```python
from build123d import *

# Parameters (mm, degrees)
SALIENTE_EXTRUIR1_DEPTH = 2.5
SALIENTE_EXTRUIR2_START = 90
SALIENTE_EXTRUIR2_DEPTH = 90
CORTAR_EXTRUIR2_REACH   = 171.292
CORTAR_EXTRUIR4_DEPTH   = 63
REDONDEO1_R             = 1
CORTAR_EXTRUIR5_REACH   = 171.292
CROQUIS7_R              = 1.5
CORTAR_EXTRUIR6_DEPTH   = 5


with BuildPart() as part:
    # Croquis1 → Saliente-Extruir1 (new body)
    with BuildSketch(Plane(origin=(0, 95.6, 0), x_dir=(1, 0, 0), z_dir=(0, 1, 0))):
        with BuildLine():
            Line((327.757359313, -46.5), (227.242640687, -46.5))
            Line((227.242640687, -46.5), (217.1, -46.5))
            ThreePointArc((217.1, -46.5), (214.271572875, -45.328427125), (213.1, -42.5))
            Line((213.1, -42.5), (213.1, 42.5))
            ThreePointArc((213.1, 42.5), (214.271572875, 45.328427125), (217.1, 46.5))
            Line((217.1, 46.5), (227.242640687, 46.5))
            Line((227.242640687, 46.5), (327.757359313, 46.5))
            ThreePointArc((327.757359313, 46.5), (331.966877069, 45.662674858), (335.535533906, 43.278174593))
            Line((335.535533906, 43.278174593), (339.778174891, 39.035533608))
            ThreePointArc((339.778174891, 39.035533608), (342.162674938, 35.466876874), (343, 31.257359313))
            Line((343, 31.257359313), (343, -31.257359312))
            ThreePointArc((343, -31.257359312), (342.162674858, -35.466877069), (339.778174593, -39.035533906))
            Line((339.778174593, -39.035533906), (335.535533608, -43.278174891))
            ThreePointArc((335.535533608, -43.278174891), (331.966876874, -45.662674939), (327.757359313, -46.5))
        make_face()
    extrude(amount=SALIENTE_EXTRUIR1_DEPTH)

    # Croquis2 → Saliente-Extruir2 (add)
    with BuildSketch(Plane.XZ.offset(-95.6).offset(SALIENTE_EXTRUIR2_START)):
        with BuildLine():
            Line((213.1, 42.5), (213.1, -42.5))
            ThreePointArc((213.1, -42.5), (214.271572875, -45.328427125), (217.1, -46.5))
            Line((217.1, -46.5), (327.757359313, -46.5))
            ThreePointArc((327.757359313, -46.5), (331.966877069, -45.662674858), (335.535533906, -43.278174593))
            Line((335.535533906, -43.278174593), (339.778174891, -39.035533608))
            ThreePointArc((339.778174891, -39.035533608), (342.162674938, -35.466876874), (343, -31.257359313))
            Line((343, -31.257359313), (343, 31.257359312))
            ThreePointArc((343, 31.257359312), (342.162674858, 35.466877069), (339.778174593, 39.035533906))
            Line((339.778174593, 39.035533906), (335.535533608, 43.278174891))
            ThreePointArc((335.535533608, 43.278174891), (331.966876874, 45.662674939), (327.757359313, 46.5))
            Line((327.757359313, 46.5), (217.1, 46.5))
            ThreePointArc((217.1, 46.5), (214.271572875, 45.328427125), (213.1, 42.5))
        make_face()
        with BuildLine():
            Line((220.6, 39), (220.6, -39))
            Line((220.6, -39), (327.757359313, -39))
            ThreePointArc((327.757359313, -39), (329.096751326, -38.733578364), (330.232233047, -37.974873734))
            Line((330.232233047, -37.974873734), (334.474874032, -33.732232749))
            ThreePointArc((334.474874032, -33.732232749), (335.233578444, -32.596751131), (335.5, -31.257359313))
            Line((335.5, -31.257359313), (335.5, 31.257359312))
            ThreePointArc((335.5, 31.257359312), (335.233578364, 32.596751326), (334.474873734, 33.732233047))
            Line((334.474873734, 33.732233047), (330.232232749, 37.974874033))
            ThreePointArc((330.232232749, 37.974874033), (329.096751131, 38.733578445), (327.757359313, 39))
            Line((327.757359313, 39), (220.6, 39))
        make_face(mode=Mode.SUBTRACT)
    extrude(amount=-SALIENTE_EXTRUIR2_DEPTH)

    # Croquis3 → Cortar-Extruir2 (cut, up to next)
    with BuildSketch(Plane(origin=(343, 0, 0), x_dir=(0, 0, -1), z_dir=(1, 0, 0)), mode=Mode.PRIVATE) as cortar_extruir2_sk1:
        with BuildLine():
            Line((23, 85.4), (-24.5, 85.4))
            ThreePointArc((-24.5, 85.4), (-27.540559159, 84.140559159), (-28.8, 81.1))
            Line((-28.8, 81.1), (-28.8, 40.6))
            ThreePointArc((-28.8, 40.6), (-27.101219331, 36.498780669), (-23, 34.8))
            Line((-23, 34.8), (24.5, 34.8))
            ThreePointArc((24.5, 34.8), (27.540559159, 36.059440841), (28.8, 39.1))
            Line((28.8, 39.1), (28.8, 79.6))
            ThreePointArc((28.8, 79.6), (27.101219331, 83.701219331), (23, 85.4))
        make_face()
    cortar_extruir2_tool1 = extrude(cortar_extruir2_sk1.sketch, amount=-CORTAR_EXTRUIR2_REACH, mode=Mode.PRIVATE) & part.part
    add(cortar_extruir2_tool1.solids().sort_by_distance((343, 60.1, 0))[0], mode=Mode.SUBTRACT)

    # Croquis4 → Cortar-Extruir4 (cut)
    with BuildSketch(Plane(origin=(0, 98.1, 0), x_dir=(1, 0, 0), z_dir=(0, 1, 0))):
        Polygon((232.757359313, -33.9), (232.757359313, -38.5), (232.757359313, -46.5), (326.657359313, -46.5), (326.657359313, -38.5), (326.657359313, -33.9), align=None)
        Polygon((326.657359313, 46.5), (232.757359313, 46.5), (232.757359313, 38.5), (232.757359313, 33.9), (326.657359313, 33.9), (326.657359313, 38.5), align=None)
    extrude(amount=-CORTAR_EXTRUIR4_DEPTH, mode=Mode.SUBTRACT)

    # Redondeo1
    redondeo1_edges = [part.edges().sort_by_distance(p)[0] for p in [
        (232.757359313, 95.6, -36.45),
        (279.707359313, 95.6, -33.9),
        (326.657359313, 95.6, -36.45),
        (279.707359313, 95.6, 33.9),
        (232.757359313, 95.6, 36.45),
        (326.657359313, 95.6, 36.45),
        (279.707359313, 35.1, 39),
        (279.707359313, 35.1, -39),
        (326.657359313, 65.35, 39),
        (232.757359313, 65.35, 39),
        (232.757359313, 96.85, 33.9),
        (326.657359313, 96.85, 33.9),
        (326.657359313, 35.1, 42.75),
        (279.707359313, 35.1, 46.5),
        (326.657359313, 66.6, 46.5),
        (232.757359313, 35.1, 42.75),
        (232.757359313, 66.6, 46.5),
        (326.657359313, 98.1, 40.2),
        (279.707359313, 98.1, 33.9),
        (232.757359313, 98.1, 40.2),
        (326.657359313, 65.35, -39),
        (326.657359313, 96.85, -33.9),
        (232.757359313, 65.35, -39),
        (326.657359313, 35.1, -42.75),
        (326.657359313, 66.6, -46.5),
        (232.757359313, 96.85, -33.9),
        (232.757359313, 35.1, -42.75),
        (279.707359313, 35.1, -46.5),
        (232.757359313, 66.6, -46.5),
        (326.657359313, 98.1, -40.2),
        (232.757359313, 98.1, -40.2),
        (279.707359313, 98.1, -33.9),
    ]]
    fillet(redondeo1_edges, radius=REDONDEO1_R)

    # Croquis5 → Cortar-Extruir5 (cut, up to next)
    with BuildSketch(Plane.ZY.offset(-213.1), mode=Mode.PRIVATE) as cortar_extruir5_sk1:
        with BuildLine():
            Line((-19.675765155, 71.72423484), (-19.675765155, 48.475765161))
            ThreePointArc((-19.675765155, 48.475765161), (-21.433124468, 44.233124467), (-25.675765163, 42.475765155))
            Line((-25.675765163, 42.475765155), (-31.024234836, 42.475765155))
            ThreePointArc((-31.024234836, 42.475765155), (-35.266875531, 44.233124467), (-37.024234845, 48.475765162))
            Line((-37.024234845, 48.475765162), (-37.024234845, 71.724234837))
            ThreePointArc((-37.024234845, 71.724234837), (-35.266875532, 75.966875532), (-31.024234837, 77.724234845))
            Line((-31.024234837, 77.724234845), (-25.675765164, 77.724234845))
            ThreePointArc((-25.675765164, 77.724234845), (-21.433124469, 75.966875534), (-19.675765155, 71.72423484))
        make_face()
    cortar_extruir5_tool1 = extrude(cortar_extruir5_sk1.sketch, amount=-CORTAR_EXTRUIR5_REACH, mode=Mode.PRIVATE) & part.part
    add(cortar_extruir5_tool1.solids().sort_by_distance((213.1, 60.1, -28.35))[0], mode=Mode.SUBTRACT)

    # Croquis7 → Cortar-Extruir6 (cut)
    with BuildSketch(Plane(origin=(0, 98.1, 0), x_dir=(1, 0, 0), z_dir=(0, 1, 0))):
        with Locations(Location((321.080026167, 18.000457457, 0), (0, 0, 270))):
            Circle(CROQUIS7_R)
        with Locations(Location((321.080026167, -18.000457457, 0), (0, 0, 270))):
            Circle(CROQUIS7_R)
    extrude(amount=-CORTAR_EXTRUIR6_DEPTH, mode=Mode.SUBTRACT)


solid = part.part
```
Design review of the part built by this model. Coordinates are the model's own, in mm. A direction names the side the tool comes from. Coordinates: 2 decimals unless noted, no trailing zeros. Loops run counter-clockwise (first coordinate to the right, second up) from the corner with the lowest first, then second, coordinate; pieces in that order, holes last.
Q1. Tool access review of faces 4 (the face through (339.3, 36.03, -27.51)), 5 (the face through (263, 30, 39)), 6 (the face through (216.797, 76.013, -21.48)): name each direction out of +Z, -Z, +X, -X, +Y, -Y from which nothing blocks a thin tool from reaching the whole face with its end or side.
Reported:
face 4: +X
face 5: -Y
face 6: +X, -X
Q2. For pin 1 (1.6 mm diameter, centred on x = 291.5, z = -43, fed in from +Y); pin 2 (10 mm diameter, centred on x = 322.5, y = 36, fed in from +Z); pin 3 (5 mm diameter, centred on x = 299.5, z = -23, fed in from -Y); pin 4 (1 mm diameter, centred on y = 38.5, z = -10, fed in from +X), all flat-tipped, find the tip position at first contact; note any pin that passes through.
Reported:
pin 1: stops at y = 35.1
pin 2: stops at z = 46.5
pin 3: stops at y = 95.6
pin 4: stops at x = 220.6
Q3. We need section A-A on z = 5. State the section outline as (x, y) points, and give its area (3 significant figures).
Reported:
outline: (213.1, 5.6) - (220.6, 5.6) - (220.6, 95.6) - (335.5, 95.6) - (335.5, 85.4) - (343, 85.4) - (343, 98.1) - (213.1, 98.1) - close; (335.5, 5.6) - (343, 5.6) - (343, 34.8) - (335.5, 34.8) - close
area: 1,300 mm2
Q4. We need section C-C on y = 18.5. State the section outline as (x, z) points.
Reported:
outline: (213.1, -42.5) arc R4 ccw to (217.1, -46.5) - (327.76, -46.5) arc R11 ccw to (335.54, -43.28) - (339.78, -39.04) arc R11 ccw to (343, -31.26) - (343, 31.26) arc R11 ccw to (339.78, 39.04) - (335.54, 43.28) arc R11 ccw to (327.76, 46.5) - (217.1, 46.5) arc R4 ccw to (213.1, 42.5) - close; hole (220.6, -39) - (327.76, -39) arc R3.5 ccw to (330.23, -37.97) - (334.47, -33.73) arc R3.5 ccw to (335.5, -31.26) - (335.5, 31.26) arc R3.5 ccw to (334.47, 33.73) - (330.23, 37.97) arc R3.5 ccw to (327.76, 39) - (220.6, 39) - close
Q5. To check wall thickness, follow line 1 (X direction, y = 29, z = -27); line 2 (Z direction, x = 266, y = 19); line 3 (Y direction, x = 336, z = -2). State the ranges of each line that lie inside material, in increasing order.
Reported:
line 1: x = 213.1 to 220.6, 335.5 to 343
line 2: z = -46.5 to -39, 39 to 46.5
line 3: y = 5.6 to 34.8, 85.4 to 98.1
Q6. We need section B-B on x = 312. State the section outline as (y, z) points.
Reported:
outline: (5.6, -46.5) - (34.1, -46.5) arc R1 ccw to (35.1, -45.5) - (35.1, -40) arc R1 ccw to (34.1, -39) - (5.6, -39) - close; (5.6, 39) - (34.1, 39) arc R1 ccw to (35.1, 40) - (35.1, 45.5) arc R1 ccw to (34.1, 46.5) - (5.6, 46.5) - close; (95.6, -32.9) arc R1 ccw to (96.6, -33.9) - (97.1, -33.9) arc R1 ccw to (98.1, -32.9) - (98.1, 32.9) arc R1 ccw to (97.1, 33.9) - (96.6, 33.9) arc R1 ccw to (95.6, 32.9) - close
Q7. The part is to be moulded in two halves that separate along X. For faces 1 (the face through (335.5, 30, 0)), 2 (the face through (216.797, 44.187, -35.22)), 3 (the face through (337.627, 51.202, -41.187)), say which applies: +X half, -X half, draft (parallel to the pull), parting line (faces both ways), or undercut.
Reported:
face 1: undercut
face 2: draft
face 3: +X half
Q8. We need section D-D on z = -18. State the section outline as (x, y) points, and give its area (3 significant figures).
Reported:
outline: (213.1, 5.6) - (220.6, 5.6) - (220.6, 95.6) - (319.58, 95.6) - (319.58, 98.1) - (213.1, 98.1) - close; (322.58, 95.6) - (335.5, 95.6) - (335.5, 85.4) - (343, 85.4) - (343, 98.1) - (322.58, 98.1) - close; (335.5, 5.6) - (343, 5.6) - (343, 34.8) - (335.5, 34.8) - close
area: 1,290 mm2
